from build123d import *

# Parameters (mm, degrees)
SKETCH2_W               = 17.3355
SKETCH2_H               = 14.351
BOSS_EXTRUDE1_DEPTH     = 6.1722
SKETCH3_W               = 17.3355
SKETCH3_H               = 12.4714
BOSS_EXTRUDE2_DEPTH     = 12.0142
SKETCH4_R               = 1.1938
BOSS_EXTRUDE3_DEPTH     = 0.381
LPATTERN1_COUNT         = 2
LPATTERN1_PITCH         = 8.8392
LPATTERN1_COL_COUNT     = 2
LPATTERN1_COL_PITCH     = 8.8392
MIRROR1_COPY_1_SKETCH_R = 1.1938
MIRROR1_COPY_1_DEPTH    = 0.381
MIRROR1_COPY_2_SKETCH_R = 1.1938
MIRROR1_COPY_2_DEPTH    = 0.381


with BuildPart() as part:
    # Sketch1 → Revolve1 (revolve)
    with BuildSketch(Plane.XY):
        with BuildLine():
            Line((0, 0), (7.0358, 0))
            ThreePointArc((7.0358, 0), (6.5659, 0.518885714), (5.8928, 0.7112))
            Line((5.8928, 0.7112), (5.8928, 12.8016))
            Line((5.8928, 12.8016), (4.0005, 12.8016))
            Line((4.0005, 12.8016), (4.0005, 17.9578))
            Line((4.0005, 17.9578), (5.04825, 17.9578))
            Line((5.04825, 17.9578), (5.04825, 22.9743))
            Line((5.04825, 22.9743), (0, 22.9743))
            Line((0, 22.9743), (0, 0))
        make_face()
    revolve(axis=Axis((0, 17.332868294, 0), (0, -1, 0)))

    # Sketch2 → Boss-Extrude1 (add)
    with BuildSketch(Plane.XZ):
        Rectangle(SKETCH2_W, SKETCH2_H)
    extrude(amount=BOSS_EXTRUDE1_DEPTH)

    # Sketch3 → Boss-Extrude2 (add)
    with BuildSketch(Plane.XZ.offset(6.1722)):
        Rectangle(SKETCH3_W, SKETCH3_H)
    extrude(amount=BOSS_EXTRUDE2_DEPTH)

    # Sketch4 → Boss-Extrude3 (add, symmetric)
    with BuildSketch(Plane(origin=(0, 0, 0), x_dir=(0, 0, -1), z_dir=(1, 0, 0))):
        with BuildLine():
            Line((6.2357, -18.1864), (9.6647, -18.1864))
            ThreePointArc((9.6647, -18.1864), (11.517333585, -14.227334736), (7.290649082, -15.3416))
            Line((7.290649082, -15.3416), (6.2357, -15.3416))
            Line((6.2357, -15.3416), (6.2357, -18.1864))
        make_face()
        with Locations((9.6647, -15.7734)):
            Circle(SKETCH4_R, mode=Mode.SUBTRACT)
    boss_extrude3 = extrude(amount=BOSS_EXTRUDE3_DEPTH, both=True)

    # LPattern1: Boss-Extrude3 ×2
    with Locations(*[(i * LPATTERN1_PITCH, 0, 0) for i in range(1, LPATTERN1_COUNT)]):
        add(boss_extrude3)

    # LPattern1 col: Boss-Extrude3 ×2
    with Locations(*[(-i * LPATTERN1_COL_PITCH, 0, 0) for i in range(1, LPATTERN1_COL_COUNT)]):
        add(boss_extrude3)

    # Mirror1: Boss-Extrude3 across plane
    add(boss_extrude3.mirror(Plane.XY))

    # Mirror1 copy 1 sketch → Mirror1 copy 1 (add, symmetric)
    with BuildSketch(Plane(origin=(8.8392, 0, 0), x_dir=(0, 0, 1), z_dir=(1, 0, 0))):
        with BuildLine():
            Line((6.2357, 18.1864), (9.6647, 18.1864))
            ThreePointArc((9.6647, 18.1864), (11.517333585, 14.227334736), (7.290649082, 15.3416))
            Line((7.290649082, 15.3416), (6.2357, 15.3416))
            Line((6.2357, 15.3416), (6.2357, 18.1864))
        make_face()
        with Locations((9.6647, 15.7734)):
            Circle(MIRROR1_COPY_1_SKETCH_R, mode=Mode.SUBTRACT)
    extrude(amount=MIRROR1_COPY_1_DEPTH, both=True)

    # Mirror1 copy 2 sketch → Mirror1 copy 2 (add, symmetric)
    with BuildSketch(Plane(origin=(-8.8392, 0, 0), x_dir=(0, 0, 1), z_dir=(1, 0, 0))):
        with BuildLine():
            Line((6.2357, 18.1864), (9.6647, 18.1864))
            ThreePointArc((9.6647, 18.1864), (11.517333585, 14.227334736), (7.290649082, 15.3416))
            Line((7.290649082, 15.3416), (6.2357, 15.3416))
            Line((6.2357, 15.3416), (6.2357, 18.1864))
        make_face()
        with Locations((9.6647, 15.7734)):
            Circle(MIRROR1_COPY_2_SKETCH_R, mode=Mode.SUBTRACT)
    extrude(amount=MIRROR1_COPY_2_DEPTH, both=True)


solid = part.part
Part model, mm, in its own coordinate system. A direction names the side the tool comes from. Coordinates: 2 decimals unless noted, no trailing zeros. Order: outer loops, then holes, each group sorted by start corner. A loop starts at its lowest first (then second) coordinate and runs counter-clockwise, first axis right, second up.
(1) Pull direction Z, two halves, no side cores. Call faces 1 (the face through (0, -3, 7.176)), 2 (the face through (8.84, -14.29, 11.57)), 3 (the face through (0, 22.974, 0)), 4 (the face through (-1.09, 20.5, -4.93)): pulls with the +Z half, pulls with the -Z half, needs draft (parallel to the pull), parting line crosses it, or undercut.
Check sheet entries:
face 1: pulls with the +Z half
face 2: undercut
face 3: needs draft
face 4: parting line crosses it
(2) Tool access for faces 5 (the face through (-0.381, -16, 8)), 6 (the face through (-0.381, -16, -8)), 7 (the face through (5.62, 6.84, 1.77)), 8 (the face through (-0.9, 15.4, -3.9)), 9 (the face through (8.834, -16.231, -10.767)): list every direction of +Z, -Z, +X, -X, +Y, -Y with a clear straight run to the whole face (end or side of a thin tool).
Check sheet entries:
face 5: +Z, -Y
face 6: -Z, -Y
face 7: +Y
face 8: none
face 9: +X, -X
(3) Slice it at D-D, the plane y = 13.5. Write the cut outline in (x, z).
Check sheet entries:
outline: circle Ø8 at (0, 0)
(4) Slice it at C-C, the plane y = 8.5. Write the cut outline in (x, z).
Check sheet entries:
outline: circle Ø11.79 at (0, 0)
(5) Probe L1, parallel to Y at x = -3, z = -3; L2, parallel to Y at x = 8.5, z = 4; L3, parallel to Z at x = 3.5, y = -15.5. List the from-to ranges inside material, lowest first.
Check sheet entries:
L1: y = -18.19 to 12.8, 17.96 to 22.97
L2: y = -18.19 to 0
L3: z = -6.24 to 6.24
(6) Slice it at A-A, the plane x = 7.5. Write the cut outline in (y, z).
Check sheet entries:
outline: (-18.19, -6.24) - (-6.17, -6.24) - (-6.17, -7.18) - (0, -7.18) - (0, 7.18) - (-6.17, 7.18) - (-6.17, 6.24) - (-18.19, 6.24) - close
(7) Slice it at B-B, the plane z = 0. Write the cut outline in (x, y), and give its area (3 significant figures).
Check sheet entries:
outline: (-8.67, -18.19) - (8.67, -18.19) - (8.67, 0) - (7.04, 0) arc R1.27 ccw to (5.89, 0.71) - (5.89, 12.8) - (4, 12.8) - (4, 17.96) - (5.05, 17.96) - (5.05, 22.97) - (-5.05, 22.97) - (-5.05, 17.96) - (-4, 17.96) - (-4, 12.8) - (-5.89, 12.8) - (-5.89, 0.71) arc R1.27 ccw to (-7.04, 0) - (-8.67, 0) - close
area: 559 mm2
(8) Pin check, flat tips, straight feed: pin 1 Ø1.9 at (x, y) = (3.5, -3) entering from -Z; pin 2 Ø8 at (y, z) = (14.5, -5.5) entering from +X; pin 3 Ø2 at (y, z) = (5, 0.5) entering from +X. Stop position of each tip, or through.
Check sheet entries:
pin 1: stops at z = -7.18
pin 2: stops at x = 5.59
pin 3: stops at x = 5.89
